Read the model definition and answer for the solid it produces. Units are mm, in the model's axes. Coordinates: 2 decimals unless noted, no trailing zeros. Loops run counter-clockwise (first coordinate to the right, second up) from the corner with the lowest first, then second, coordinate; pieces in that order, holes last.
Autodesk Inventor part; units mm, degrees
ref_plane "YZ Plane" through (0, 0, 0) normal (1, 0, 0) x (0, 1, 0)
ref_plane "XZ Plane" through (0, 0, 0) normal (0, 1, 0) x (-1, 0, 0)
ref_plane "XY Plane" through (0, 0, 0) normal (0, 0, 1) x (1, 0, 0)
sketch "Sketch1" plane through (0, 0, 0) normal (1, 0, 0) x (0, 1, 0)
  line L0 (-3.6662, -6.35) -> (-7.3323, 0)
  line L1 (-7.3323, 0) -> (-3.6662, 6.35)
  line L2 (-3.6662, 6.35) -> (3.6662, 6.35)
  line L3 (3.6662, 6.35) -> (7.3323, 0)
  line L4 (7.3323, 0) -> (3.6662, -6.35)
  line L5 (3.6662, -6.35) -> (-3.6662, -6.35)
  point P0 (0, 0)
  point P1 (0, 0)
  dimension "d0" = 12.7
extrude "Extrusion1" add sketch "Sketch1" along normal blind 207.1878
sketch "Sketch2" plane through (0, 0, 0) normal (-1, 0, 0) x (0, 0, 1)
  point P0 (0, 0)
  point P1 (0, 0)
hole "Hole1" at (0, 0, 0) direction (1, 0, 0) diameter 3.9624 depth 31.75 tip angle 118
sketch "Sketch3" plane through (207.1878, 0, 0) normal (1, 0, 0) x (0, 0, -1)
  circle A0 centre (0, 0) radius 1.9812
hole "Hole2" at (207.1878, 0, 0) direction (-1, 0, 0) diameter 3.9624 depth 31.75 tip angle 118
properties part number "STOCK,HEX,SHAFT,KICKER,BACK"
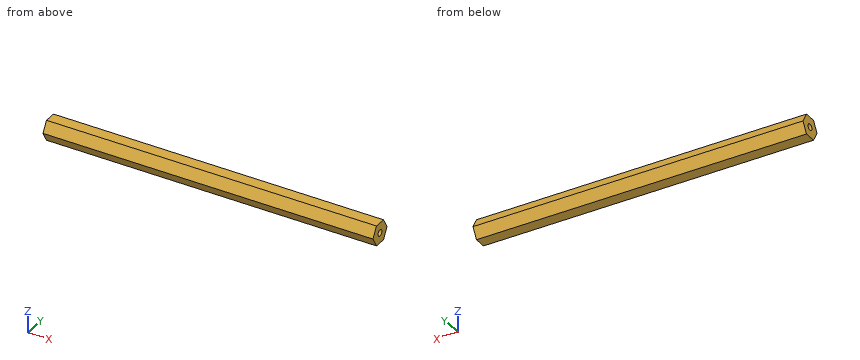
Q1. A cutting plane is placed at B-B (z = -4.25). Give the vertices of the cut face in (x, y), then the cut area to 3 significant figures.
Findings below:
outline: (0, -4.88) - (207.19, -4.88) - (207.19, 4.88) - (0, 4.88) - close
area: 2,020 mm2
Q2. Straight lines are drawn through the part: probe 1 along Z at (x, y) = (200, 0); probe 2 along Y at (x, z) = (10, 0); probe 3 along X at (y, z) = (1.25, -1.5). For each, find the intervals that lie inside material, in ascending order.
Findings below:
probe 1: z = -6.35 to -1.98, 1.98 to 6.35
probe 2: y = -7.33 to -1.98, 1.98 to 7.33
probe 3: x = 31.77 to 175.42
Q3. A cutting plane is placed at A-A (x = 78). Give the vertices of the cut face in (y, z), then the cut area to 3 significant figures.
Findings below:
outline: (-7.33, 0) - (-3.67, -6.35) - (3.67, -6.35) - (7.33, 0) - (3.67, 6.35) - (-3.67, 6.35) - close
area: 140 mm2
Q4. A flat-ended cylindrical pin translates along its axis: pin 1 Ø1 at (x, y) = (109, 4.5) entering from +Z. Find the tip coordinate at first contact, or state that the pin passes through.
Findings below:
pin 1: stops at z = 5.77
